from build123d import *

# Parameters (mm, degrees)
F0_W     = 63.119
F0_H     = 63.627
F1_DEPTH = 118.6434
F2_W     = 25.4
F2_H     = 25.4
F3_DEPTH = 63.119
F4_R     = 3.2639
F5_DEPTH = 63.627
F6_R     = 7.9375
F7_DEPTH = 1.5494


# Not quite as in the source:
# - a feature names something its author has since deleted; it is built from what else it names


with BuildPart() as f1:
    # F0 (on Front) → F1 (new body)
    with BuildSketch(Plane.XZ):
        with Locations((-8.3619841438, 9.8403063603)):
            Rectangle(F0_W, F0_H)
    extrude(amount=F1_DEPTH)

    # F2 (on face) → F3 (cut, through all)
    with BuildSketch(Plane.YZ.offset(23.1975158562)):
        with Locations((-12.7, -9.2731936397)):
            Rectangle(F2_W, F2_H)
    extrude(amount=-F3_DEPTH, mode=Mode.SUBTRACT)

    # F4 (on face) → F5 (cut, through all)
    with BuildSketch(Plane(origin=(0, 0, -21.9731936397), x_dir=(1, 0, 0), z_dir=(0, 0, -1))):
        with Locations((7.7937371098, 106.303319335)):
            Circle(F4_R)
    extrude(amount=-F5_DEPTH, mode=Mode.SUBTRACT)

    # F6 (on face) → F7 (cut)
    with BuildSketch(Plane(origin=(0, 0, -21.9731936397), x_dir=(1, 0, 0), z_dir=(0, 0, -1))):
        with Locations((7.7937371098, 106.303319335)):
            Circle(F6_R)
    extrude(amount=-F7_DEPTH, mode=Mode.SUBTRACT)


solid = f1.part
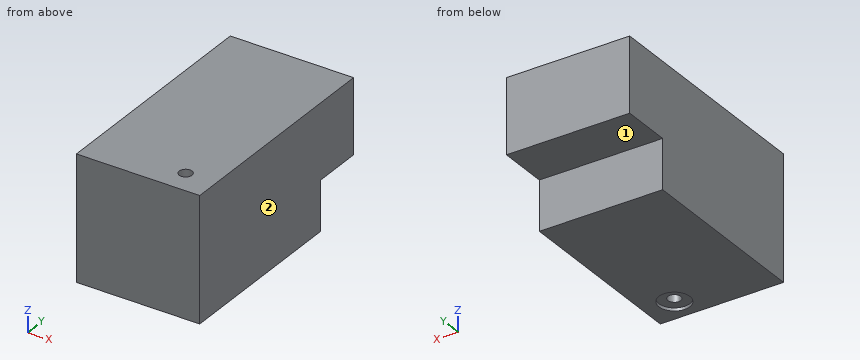
Could you check a few things on this model? Use its own coordinates, in mm. Face numbers are marked on the shaded views. A direction names the side the tool comes from. Coordinates: 2 decimals unless noted, no trailing zeros. Write each loop counter-clockwise with the first axis right and the second up, starting at its lowest first coordinate (ties: lowest second). Pieces come first, ordered by that corner, then holes. Notation, with made-up numbers: (38.5, 40.25) - (67.5, 40.25) arc R26 ccw to (67.5, 56.25) - close; hole circle Ø4 at (-15.75, 70). An arc over 180 degrees is marked (long way). Put each result on its own line as item: value. Start each with the question number.
Q1. I want a section at B-B on z = -5. Write out the boundary of the cut face in (x, y), plus the area to 3 significant figures.
Q2. Which directions (+Z, -Z, +X, -X, +Y, -Y) give clear straight access to the entire face, cutting with the end or side of a thin tool? Please do the marked faces 1 and 2.
Q3. I'm going to push flat-ended pins straight in: P1, Ø6, axis at x = -30, z = -7.5, coming from the +Y side; P2, Ø5, axis at x = 7.5, y = -108.5, coming from the -Z side; P3, Ø7.5, axis at x = 4.5, y = -7, coming from the -Z side. Where does each tip first touch, or does it pass through?
Q4. Please list where these lines run through material, in increasing order: L1, parallel to Z at x = -22.5, y = -6; L2, parallel to Y at x = -30, z = 3.
Q5. I want a section at A-A on x = -19. Write out the boundary of the cut face in (y, z).
Checks:
1. outline: (-39.92, -118.64) - (23.2, -118.64) - (23.2, -25.4) - (-39.92, -25.4) - close; hole circle Ø6.53 at (7.79, -106.3)
1. area: 5,850 mm²
2. face 1: -Z, +X, -X, +Y
2. face 2: +Z, -Z, +X, +Y, -Y
3. P1: y = -25.4
3. P2: z = -20.42
3. P3: z = 3.43
4. L1: 3.43 to 41.65
4. L2: -118.64 to -25.4
5. outline: (-118.64, -21.97) - (-25.4, -21.97) - (-25.4, 3.43) - (0, 3.43) - (0, 41.65) - (-118.64, 41.65) - close
